Geometry: final body of the model. Coordinates: model frame, mm. A direction names the side the tool comes from. Give positions to 0.01 mm unless a question says otherwise; leave off trailing zeros. Write each loop counter-clockwise with the first axis right and the second up, starting at its lowest first coordinate (ties: lowest second). Pieces come first, ordered by that corner, then holes. Notation, with made-up numbers: M -37,-29.5 L -1,-29.5 A10 ccw -1,-23.5 Z; hole C 68.25,-26.5 d2. An arc over 180 degrees is marked long. Answer as a JSON object with one key per item and string values.
Autodesk Inventor part; units mm, degrees
ref_plane "YZ Plane" through (0, 0, 0) normal (1, 0, 0) x (0, 1, 0)
ref_plane "XZ Plane" through (0, 0, 0) normal (0, 1, 0) x (-1, 0, 0)
ref_plane "XY Plane" through (0, 0, 0) normal (0, 0, 1) x (1, 0, 0)
sketch "Schizzo1" plane through (0, 0, 0) normal (0, 0, 1) x (1, 0, 0)
  line L0 (-18.5, 30) -> (-18.5, 0)
  line L1 (-18.5, 0) -> (18.5, 0)
  line L2 (18.5, 0) -> (18.5, 30)
  line L3 (18.5, 30) -> (13.5, 30)
  line L4 (13.5, 30) -> (13.5, 5)
  line L5 (13.5, 5) -> (-13.5, 5)
  line L6 (-13.5, 5) -> (-13.5, 30)
  line L7 (-13.5, 30) -> (-18.5, 30)
  point P0 (0, 0)
  point P1 (0, 5)
  point P2 (0, 0)
  dimension "d0" = 37
  dimension "d1" = 27
  dimension "d2" = 5
  dimension "d3" = 30
extrude "Estrusione1" add sketch "Schizzo1" along normal blind 15
sketch "Schizzo2" plane through (0, 0, 0) normal (1, 0, 0) x (0, 1, 0)
  line L0 (5, 0) -> (30, 0)
  line L1 (30, 0) -> (30, 15)
  line L2 (5, 15) -> (30, 15)
  line L3 (5, 0) -> (5, 15)
  circle A0 centre (20, 7.5) radius 5
  point P0 (0, 0)
  point P1 (30, 7.5)
  point P2 (17.5, 0)
  dimension "d6" = 10
  dimension "d23" = 10
extrude "Estrusione2" cut sketch "Schizzo2" along normal through all both and the other way through all contours A0
fillet "Raccordo1" radius 2 6 edges at (-16, 30, 15) (-16, 30, 0) (16, 30, 15) (16, 30, 0) (18.5, 0, 7.5) (-18.5, 0, 7.5)
sketch "Schizzo3" plane through (-16.5, 0, 0) normal (0, -1, 0) x (1, 0, 0)
  line L0 (0, 0) -> (0, 15)
  line L1 (0, 0) -> (33, 0)
  line L2 (33, 15) -> (33, 0)
  line L3 (0, 15) -> (33, 15)
  circle A0 centre (16.5, 7.5) radius 6
  point P0 (16.5, 0)
  point P1 (33, 7.5)
  point P2 (16.5, 0)
  dimension "d13" = 12
extrude "Estrusione3" add sketch "Schizzo3" along normal blind 5 contours A0
sketch "Schizzo4" plane through (0, -5, 7.5) normal (0, -1, 0) x (1, 0, 0)
  circle A0 centre (0, 0) radius 3
  point P0 (0, -7.5)
  dimension "d16" = 6
extrude "Estrusione4" add sketch "Schizzo4" along normal blind 12
chamfer "Smusso1" distance 0.5 angle 45 6 edges at (-13.5, 15, 7.5) (13.5, 15, 7.5) (-18.5, 15, 7.5) (18.5, 15, 7.5) (-3, -17, 7.5) (-6, -5, 7.5)
thread "Filettatura2"
properties part number "Forcella movimento lama" material "Acciaio inossidabile"
1) Pull-direction query (Y, two-part tool) for faces 4 (the flat face through (-18.5, 13, 7)), 5 (the cylindrical face through (15.96, 29.4, 14.43)), 6 (the cylindrical face through (-15.972, 19.349, 12.457)); classes: pulls with the +Y half, pulls with the -Y half, needs draft (parallel to the pull), parting line crosses it, or undercut.
Geometry check:
{"face 4": "needs draft", "face 5": "pulls with the +Y half", "face 6": "undercut"}
2) Cut plane B-B on z = 7.5. Give the number of separate pieces and of enclosed holes in the cut face, and give its area (3 significant figures).
Geometry check:
{"separate pieces": "3", "enclosed holes": "0", "area": "464 mm2"}
3) Cut plane D-D on y = -2. Return loops of the section in (x, z), and give its area (3 significant figures).
Geometry check:
{"outline": "C 0,7.5 d12", "area": "113 mm2"}
4) Cut plane C-C on x = 0. Return loops of the section in (y, z), and give its area (4 significant figures).
Geometry check:
{"outline": "M -17,5 L -16.5,4.5 L -5,4.5 L -5,2 L -4.5,1.5 L 0,1.5 L 0,0 L 5,0 L 5,15 L 0,15 L 0,13.5 L -4.5,13.5 L -5,13 L -5,10.5 L -16.5,10.5 L -17,10 Z", "area": "206.5 mm2"}
5) Set-up query: faces 1 (the flat face through (18.5, 13, 7)), 2 (the flat face through (13.5, 15, 4)), 3 (the cylindrical face through (-4.42, -2.22, 3.44)). Return all of +Z, -Z, +X, -X, +Y, -Y with unobstructed straight access to the full face (end or side cutting, diameter ignored); none if empty.
Geometry check:
{"face 1": "+Z, -Z, +X, +Y, -Y", "face 2": "+Z, -Z, +Y", "face 3": "-Y"}
6) Contact query for flat-ended pins moving along their axis: P1, Ø1.5, axis at y = 22, z = 9, coming from the +X side; P2, Ø6, axis at x = 0.5, z = 8, coming from the +Y side; P3, Ø4, axis at y = -7.5, z = 5.5, coming from the +X side; P4, Ø4.5, axis at x = 6, z = 9, coming from the -Y side. Output: stop coordinate, or through.
Geometry check:
{"P1": "passes through", "P2": "stops at y = 5", "P3": "stops at x = 3", "P4": "stops at y = -5"}
7) Line query: line 1 (Z direction, x = -14.85, y = 20); line 2 (Y direction, x = 16.55, z = 7.5); line 3 (X direction, y = 25, z = 1.75). Output: solid intervals per line, ascending. Write a range as from..to.
Geometry check:
{"line 1": "z = 0..2.5, 12.5..15", "line 2": "y = 0..15, 25..30", "line 3": "x = -18.5..-13.5, 13.5..18.5"}
8) Cut plane A-A on y = 20. Return loops of the section in (x, z), and give its area (3 significant figures).
Geometry check:
{"outline": "M -18.5,0 L -13.5,0 L -13.5,2 L -14,2.5 L -18,2.5 L -18.5,2 Z; M -18.5,13 L -18,12.5 L -14,12.5 L -13.5,13 L -13.5,15 L -18.5,15 Z; M 13.5,0 L 18.5,0 L 18.5,2 L 18,2.5 L 14,2.5 L 13.5,2 Z; M 13.5,13 L 14,12.5 L 18,12.5 L 18.5,13 L 18.5,15 L 13.5,15 Z", "area": "49.0 mm2"}
